Here's the drawing with two shaded views (mm, measured from the low corner). I have some questions. A direction names the side the tool comes from. Coordinates: 2 decimals unless noted, no trailing zeros. Write each loop counter-clockwise with the first axis right and the second up, starting at its lowest first coordinate (ties: lowest second). Pieces come first, ordered by that corner, then holes.
Item 1: If we section it at C-C (x = 14.5): Please give me the cut outline in (y, z).
Item 2: If we section it at B-B (y = 12): Please give me the cut outline in (x, z), then the cut area to 3 significant figures.
Item 3: For the marked faces 5 and 6, which set-ups out of +Z, -Z, +X, -X, +Y, -Y let a thin tool reach every point of the face, with its end or its side?
Item 4: We'd pull the mould along X, two halves only. Please class the marked faces 1, 2, 3 and 4: +X half, -X half, draft (parallel to the pull), parting line (faces both ways), or undercut.
Item 5: I'm going to push a flat-ended pin straight in: pin 1 Ø3 at (x, z) = (12, 4) entering from -Y. Where does the tip first touch, or does it pass through?
Item 6: If we section it at A-A (z = 11.5): Please give me the cut outline in (x, y).
Item 7: If I drill on line 1 (X direction, y = 2, z = 5.5); line 2 (Y direction, x = 2.5, z = 1.25); line 3 (Y direction, x = 1, z = 2.25), over which ranges is the centre line in solid material (lowest first)?
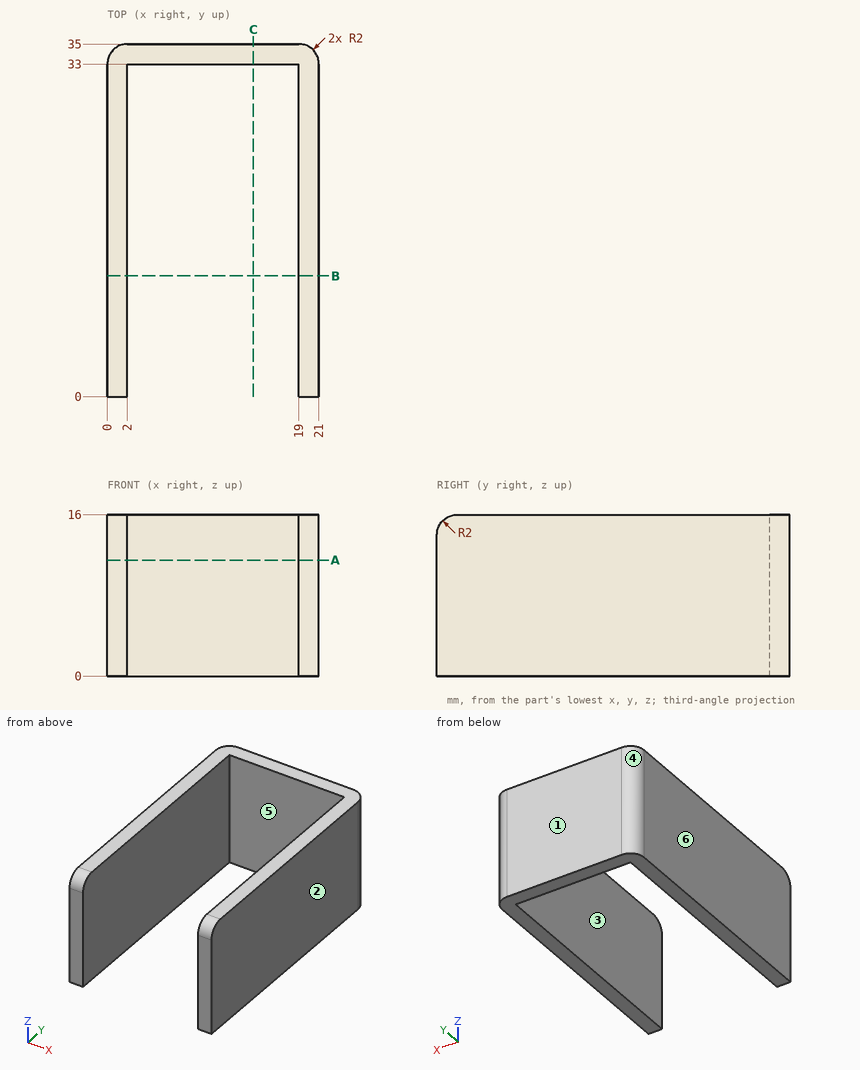
Answer list:
1. outline: (33, 0) - (35, 0) - (35, 16) - (33, 16) - close
2. outline: (0, 0) - (2, 0) - (2, 16) - (0, 16) - close; (19, 0) - (21, 0) - (21, 16) - (19, 16) - close
2. area: 64.0 mm2
3. face 5: +Z, -Z, -Y
3. face 6: +Z, -Z, -X, +Y, -Y
4. face 1: draft
4. face 2: +X half
4. face 3: undercut
4. face 4: -X half
5. pin 1: stops at y = 33
6. outline: (0, 0) - (2, 0) - (2, 33) - (19, 33) - (19, 0) - (21, 0) - (21, 33) arc R2 ccw to (19, 35) - (2, 35) arc R2 ccw to (0, 33) - close
7. line 1: x = 0 to 2, 19 to 21
7. line 2: y = 33 to 35
7. line 3: y = 0 to 34.73
